The figure shows three views and two pictorial views of one solid part (mm, origin at its lowest corner). Answer the questions. A direction names the side the tool comes from. Round coordinates to 2 decimals unless told otherwise and drop trailing zeros. Order: outer loops, then holes, each group sorted by start corner. A loop starts at its lowest first (then second) coordinate and runs counter-clockwise, first axis right, second up. Notation, with made-up numbers: (46, 23.5) -> (68, 23.5) arc R27 ccw to (68, 46.5) -> close; hole circle Ø8 at (-31.5, 39.25). An arc over 180 degrees is marked (long way). One line per item, written item: value. Start each with the question number.
1. Flat-ended cylindrical pins translate along their axes: pin 1 Ø3 at (y, z) = (39, 58) entering from -X; pin 2 Ø2 at (y, z) = (12, 71.5) entering from +X (3 decimals); pin 3 Ø21 at (x, z) = (16, 65) entering from +Y. Find the tip coordinate at first contact, or state that the pin passes through.
2. For the marked faces 1, 2 and 3, determine the directions among +Z, -Z, +X, -X, +Y, -Y from which every point of the face is accessible in a straight line to the end or side of a thin tool.
3. Consider line 1 (X direction, y = 5, z = 65); line 2 (Y direction, x = 107, z = 5.5); line 3 (X direction, y = 54, z = 40). Determine where each line is inside the solid, lowest interval first.
4. Section B-B (z = 40.5) is taken. Give the vertices of the cut face in (x, y), then the cut area to 3 significant figures.
5. The mould has two halves that part along Z. Classify the marked faces 4, 5 and 6: released by +Z, released by -Z, zero draft, split by the parting line, or undercut.
6. Section A-A (x = 64) is taken. Give the vertices of the cut face in (y, z).
7. Section D-D (x = 106.5) is taken. Give the vertices of the cut face in (y, z).
8. Section C-C (y = 7) is taken. Give the vertices of the cut face in (x, z).
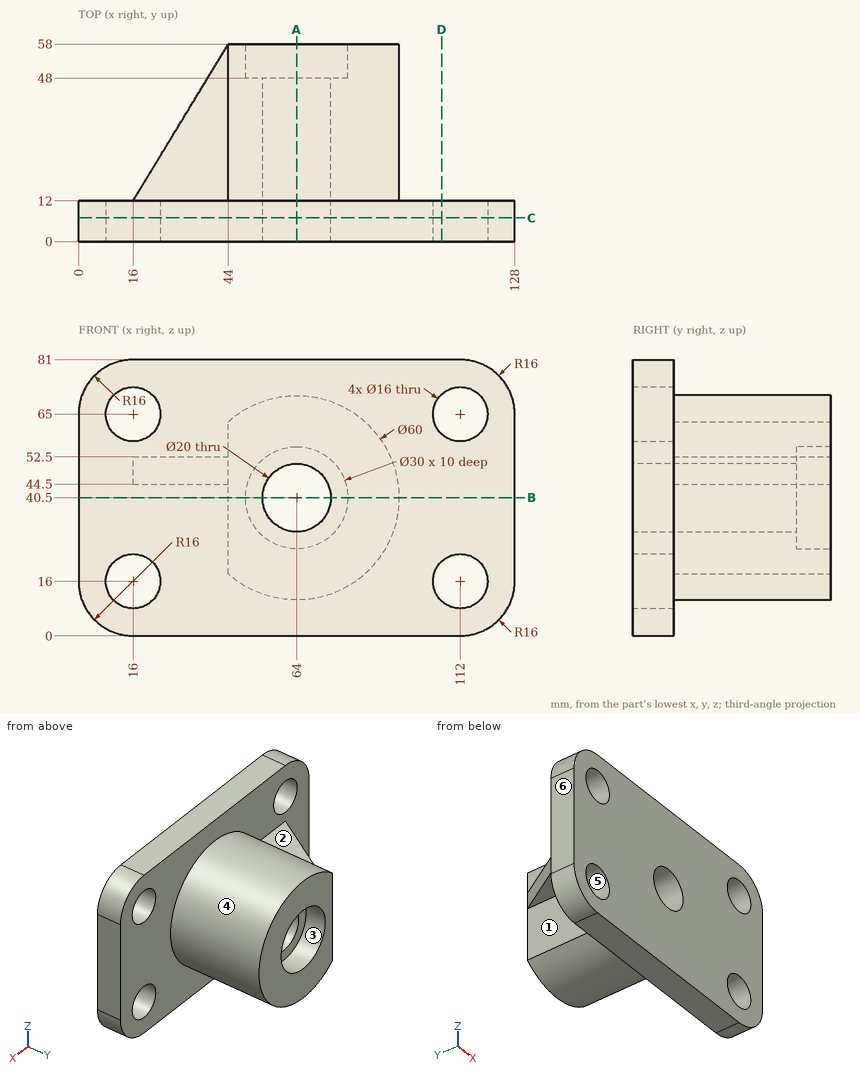
Answer:
1. pin 1: x = 44
1. pin 2: x = 127.025
1. pin 3: y = 12
2. face 1: -Z, -X, +Y
2. face 2: +Z, -X, +Y
2. face 3: +Y
3. line 1: 0 to 8, 24 to 104, 120 to 128
3. line 2: 0 to 12
3. line 3: 44 to 49.01, 78.99 to 94
4. outline: (0, 0) -> (54, 0) -> (54, 48) -> (49, 48) -> (49, 58) -> (44, 58) -> (44, 12) -> (0, 12) -> close; (74, 0) -> (128, 0) -> (128, 12) -> (94, 12) -> (94, 58) -> (79, 58) -> (79, 48) -> (74, 48) -> close
4. area: 2,580 mm^2
5. face 4: split by the parting line
5. face 5: undercut
5. face 6: zero draft
6. outline: (0, 0) -> (12, 0) -> (12, 10.5) -> (58, 10.5) -> (58, 25.5) -> (48, 25.5) -> (48, 30.5) -> (0, 30.5) -> close; (0, 50.5) -> (48, 50.5) -> (48, 55.5) -> (58, 55.5) -> (58, 70.5) -> (12, 70.5) -> (12, 81) -> (0, 81) -> close
7. outline: (0, 0) -> (12, 0) -> (12, 10.19) -> (0, 10.19) -> close; (0, 21.81) -> (12, 21.81) -> (12, 59.19) -> (0, 59.19) -> close; (0, 70.81) -> (12, 70.81) -> (12, 81) -> (0, 81) -> close
8. outline: (0, 16) arc R16 ccw to (16, 0) -> (112, 0) arc R16 ccw to (128, 16) -> (128, 65) arc R16 ccw to (112, 81) -> (16, 81) arc R16 ccw to (0, 65) -> close; hole circle Ø16 at (16, 16); hole circle Ø16 at (16, 65); hole circle Ø20 at (64, 40.5); hole circle Ø16 at (112, 16); hole circle Ø16 at (112, 65)
